Design review of the part shown in the three views and the two pictorial views. Dimensions are in mm from the part's minimum x, y and z. A direction names the side the tool comes from. Coordinates: 2 decimals unless noted, no trailing zeros. Write each loop counter-clockwise with the first axis right and the second up, starting at its lowest first coordinate (ties: lowest second). Pieces come first, ordered by that corner, then holes. Notation, with made-up numbers: (85, 35) - (105, 35) arc R15 cw to (105, 56) - close; hole circle Ø11 at (-39.75, 41.25). An arc over 180 degrees is marked (long way). Write each question's results on one line, items separated by ' | '.
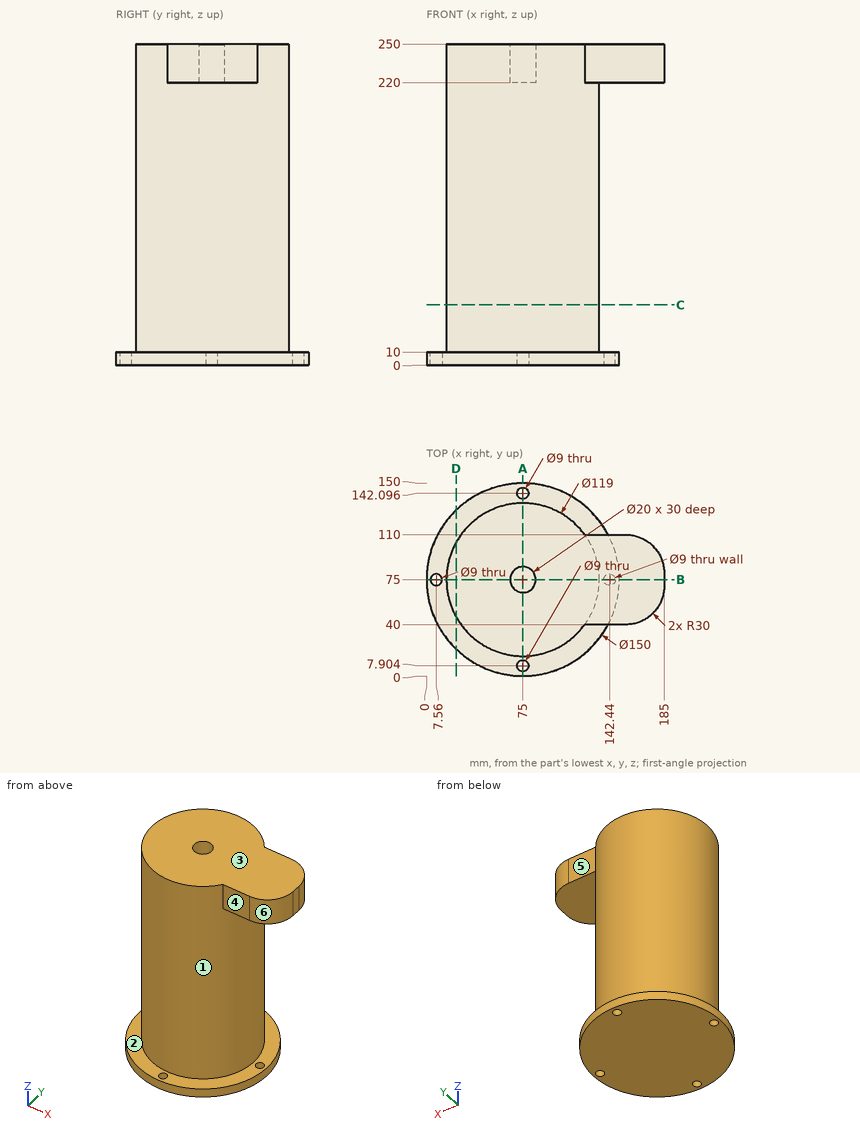
Q1. Take a section at C-C on z = 47. State the section outline as (x, y) points, plus the area to 3 significant figures.
Results found:
outline: circle Ø119 at (75, 75) | area: 11,100 mm2
Q2. Take a section at D-D on x = 23. State the section outline as (y, z) points.
Results found:
outline: (20.95, 0) - (129.05, 0) - (129.05, 10) - (103.92, 10) - (103.92, 250) - (46.08, 250) - (46.08, 10) - (20.95, 10) - close
Q3. Take a section at B-B on y = 75. State the section outline as (x, z) points, plus the area to 3 significant figures.
Results found:
outline: (0, 0) - (3.06, 0) - (3.06, 10) - (0, 10) - close; (12.06, 0) - (137.94, 0) - (137.94, 10) - (134.5, 10) - (134.5, 220) - (185, 220) - (185, 250) - (85, 250) - (85, 220) - (65, 220) - (65, 250) - (15.5, 250) - (15.5, 10) - (12.06, 10) - close; (146.94, 0) - (150, 0) - (150, 10) - (146.94, 10) - close | area: 30,800 mm2
Q4. Wall thickness on line 1 along Y through (x, z) = (75, 6); line 2 along Y through (x, z) = (75, 231); line 3 along Z through (x, y) = (136.5, 63.5): over which ranges is each line inside the solid? List them lowest first. Write a range as from..to.
Results found:
line 1: 0..3.4, 12.4..137.6, 146.6..150 | line 2: 15.5..65, 85..134.5 | line 3: 0..10, 220..250
Q5. For pin 1 (7 mm diameter, centred on x = 142.44, y = 75, fed in from -Z); pin 2 (10 mm diameter, centred on y = 68.5, z = 93.5, fed in from +X); pin 3 (10 mm diameter, centred on y = 91, z = 80, fed in from +X) (1 decimal), all flat-tipped, find the tip position at first contact; note any pin that passes through.
Results found:
pin 1: z = 220 | pin 2: x = 134.48 | pin 3: x = 133.5
Q6. Mouldability with a two-part tool opening along Z and no side actions: class the marked faces 1, 2, 3 and 4 as pulls with the +Z half, pulls with the -Z half, needs draft (parallel to the pull), parting line crosses it, or undercut.
Results found:
face 1: undercut | face 2: undercut | face 3: pulls with the +Z half | face 4: needs draft
Q7. For the marked faces 5 and 6, list the 3-axis set-ups (+Z, -Z, +X, -X, +Y, -Y) from which the entire face can be reached by the end or side of a thin tool; tool diameter is ignored.
Results found:
face 5: +Z, +X, +Y | face 6: +Z, -Z, +X, -Y
Q8. Take a section at A-A on x = 75. State the section outline as (y, z) points.
Results found:
outline: (0, 0) - (3.4, 0) - (3.4, 10) - (0, 10) - close; (12.4, 0) - (137.6, 0) - (137.6, 10) - (134.5, 10) - (134.5, 250) - (85, 250) - (85, 220) - (65, 220) - (65, 250) - (15.5, 250) - (15.5, 10) - (12.4, 10) - close; (146.6, 0) - (150, 0) - (150, 10) - (146.6, 10) - close
